```python
from build123d import *

# Parameters (mm, degrees)
SKETCH1_R               = 32.5
SKETCH1_R_2             = 20.5
BOSS_EXTRUDE1_DEPTH     = 4
SKETCH2_R               = 23.5
SKETCH2_R_2             = 20.5
BOSS_EXTRUDE2_DEPTH     = 2.5
SKETCH3_R               = 3
CUT_EXTRUDE1_DEPTH      = 1
CUT_EXTRUDE1_DEPTH_BACK = 7.5


with BuildPart() as part:
    # Sketch1 → Boss-Extrude1 (new body)
    with BuildSketch(Plane(origin=(0, 0, 0), x_dir=(1, 0, 0), z_dir=(0, 1, 0))):
        Circle(SKETCH1_R)
        Circle(SKETCH1_R_2, mode=Mode.SUBTRACT)
    extrude(amount=BOSS_EXTRUDE1_DEPTH)

    # Sketch2 → Boss-Extrude2 (add)
    with BuildSketch(Plane.XZ):
        Circle(SKETCH2_R)
        Circle(SKETCH2_R_2, mode=Mode.SUBTRACT)
    extrude(amount=BOSS_EXTRUDE2_DEPTH)

    # Sketch3 → Cut-Extrude1 (cut, two sides)
    with BuildSketch(Plane(origin=(0, 4, 0), x_dir=(1, 0, 0), z_dir=(0, 1, 0))) as cut_extrude1_sk:
        with Locations((0, 27.5)):
            Circle(SKETCH3_R)
        with Locations((23.815698604, 13.75)):
            Circle(SKETCH3_R)
        with Locations((23.815698604, -13.75)):
            Circle(SKETCH3_R)
        with Locations((0, -27.5)):
            Circle(SKETCH3_R)
        with Locations((-23.815698604, -13.75)):
            Circle(SKETCH3_R)
        with Locations((-23.815698604, 13.75)):
            Circle(SKETCH3_R)
    extrude(amount=CUT_EXTRUDE1_DEPTH, mode=Mode.SUBTRACT)
    extrude(cut_extrude1_sk.sketch, amount=-CUT_EXTRUDE1_DEPTH_BACK, mode=Mode.SUBTRACT)


solid = part.part
```
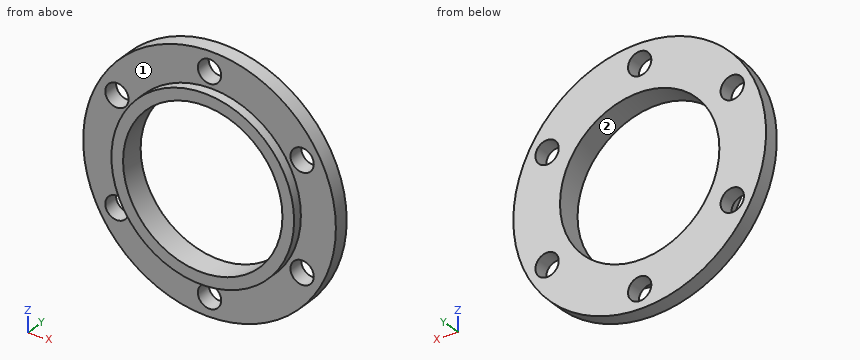
Can you work these out from the model? Positions are in its coordinate system, mm. Face numbers are marked on the shaded views. Give positions to 0.01 mm unless a question says otherwise; leave off trailing zeros. Loops run counter-clockwise (first coordinate to the right, second up) from the corner with the lowest first, then second, coordinate; pieces in that order, holes last. Notation, with made-up numbers: M 8,3 L 22,3 A6 ccw 22,10 Z; hole C 56.5,89.25 d5. An arc over 180 degrees is marked long. One line per item, written item: value.
(1) Will these pins go through, and if not, where does the flat tip stop? pin 1 (7 mm diameter, centred on x = -23.82, z = 13.75, fed in from -Y); pin 2 (1 mm diameter, centred on x = 21, y = 3, fed in from -Z).
Returned:
pin 1: y = 0
pin 2: z = -25.22
(2) I need wall thicknesses on line 1 (Z direction, x = 0, y = 3.2); line 2 (X direction, y = 2, z = 16); line 3 (X direction, y = 3, z = -15.5). Which ranges of each line are inside material? Lowest first, please.
Returned:
line 1: -32.5 to -30.5, -24.5 to -20.5, 20.5 to 24.5, 30.5 to 32.5
line 2: -28.29 to -25.8, -21.83 to -12.82, 12.82 to 21.83, 25.8 to 28.29
line 3: -28.57 to -26.25, -21.38 to -13.42, 13.42 to 21.38, 26.25 to 28.57
(3) Suppose I cut it at A-A on z = 0. List the corners of the cut face in (x, y) for me, plus the area to 3 significant figures.
Returned:
outline: M -32.5,0 L -23.5,0 L -23.5,-2.5 L -20.5,-2.5 L -20.5,4 L -32.5,4 Z; M 20.5,-2.5 L 23.5,-2.5 L 23.5,0 L 32.5,0 L 32.5,4 L 20.5,4 Z
area: 111 mm^2
(4) Suppose I cut it at C-C on x = -17. List the corners of the cut face in (y, z) for me.
Returned:
outline: M -2.5,-16.22 L 0,-16.22 L 0,-27.7 L 4,-27.7 L 4,-11.46 L -2.5,-11.46 Z; M -2.5,11.46 L 4,11.46 L 4,27.7 L 0,27.7 L 0,16.22 L -2.5,16.22 Z
(5) Suppose I cut it at D-D on z = 13. List the corners of the cut face in (x, y) for me, plus the area to 3 significant figures.
Returned:
outline: M -29.79,0 L -26.72,0 L -26.72,4 L -29.79,4 Z; M -20.91,0 L -19.58,0 L -19.58,-2.5 L -15.85,-2.5 L -15.85,4 L -20.91,4 Z; M 15.85,-2.5 L 19.58,-2.5 L 19.58,0 L 20.91,0 L 20.91,4 L 15.85,4 Z; M 26.72,0 L 29.79,0 L 29.79,4 L 26.72,4 Z
area: 83.6 mm^2
(6) Suppose I cut it at B-B on x = 0. List the corners of the cut face in (y, z) for me.
Returned:
outline: M -2.5,-23.5 L 0,-23.5 L 0,-24.5 L 4,-24.5 L 4,-20.5 L -2.5,-20.5 Z; M -2.5,20.5 L 4,20.5 L 4,24.5 L 0,24.5 L 0,23.5 L -2.5,23.5 Z; M 0,-32.5 L 4,-32.5 L 4,-30.5 L 0,-30.5 Z; M 0,30.5 L 4,30.5 L 4,32.5 L 0,32.5 Z
(7) We'd pull the mould along X, two halves only. Please class the marked faces 1 and 2: released by +X, released by -X, zero draft, split by the parting line, or undercut.
Returned:
face 1: zero draft
face 2: undercut
